Part print with two shaded views. Sizes in mm from the minimum x, y, z corner. A direction names the side the tool comes from. Give positions to 0.01 mm unless a question says otherwise; leave off trailing zeros. Write each loop counter-clockwise with the first axis right and the second up, starting at its lowest first coordinate (ties: lowest second). Pieces come first, ordered by that corner, then holes. Notation, with made-up numbers: (73.5, 71) -> (94.5, 71) arc R20 cw to (94.5, 104) -> close; hole circle Ø6 at (74, -37). An arc over 180 degrees is marked (long way). Write item = value, one per line. Start each with the question number.
Q1. Wall check: line 1 (Y direction, x = 4, z = 24.5); line 2 (Z direction, x = 14.25, y = 8); line 3 (Z direction, x = 22.25, y = 31). Give the ranges that are in metal, low to high.
Q2. Saw through at A-A, the plane x = 4. List the corners of the cut face in (y, z).
Q3. Saw through at C-C, the plane z = 4.25. List the corners of the cut face in (x, y), then the cut area to 3 significant figures.
Q4. Mould opens along Y. For the marked faces 4, 5, 6 and 7 say: pulls with the +Y half, pulls with the -Y half, needs draft (parallel to the pull), parting line crosses it, or undercut.
Q5. Tool access for the marked faces 1, 2 and 3: list every direction of +Z, -Z, +X, -X, +Y, -Y with a clear straight run to the whole face (end or side of a thin tool).
Q6. Drop flat-ended pins along their axis: P1, Ø10, axis at x = 11.5, z = 19, coming from the +Y side; P2, Ø6.5, axis at x = 8, z = 24.5, coming from the -Y side; P3, Ø8, axis at y = 14, z = 9.5, coming from the -X side; P4, Ø2, axis at x = 24.5, y = 18, coming from the -Z side. Give the stop position or say it passes through.
Q7. Saw through at B-B, the plane y = 20.5. List the corners of the cut face in (x, z).
Q8. Saw through at D-D, the plane z = 21.5. List the corners of the cut face in (x, y), then the cut area to 3 significant figures.
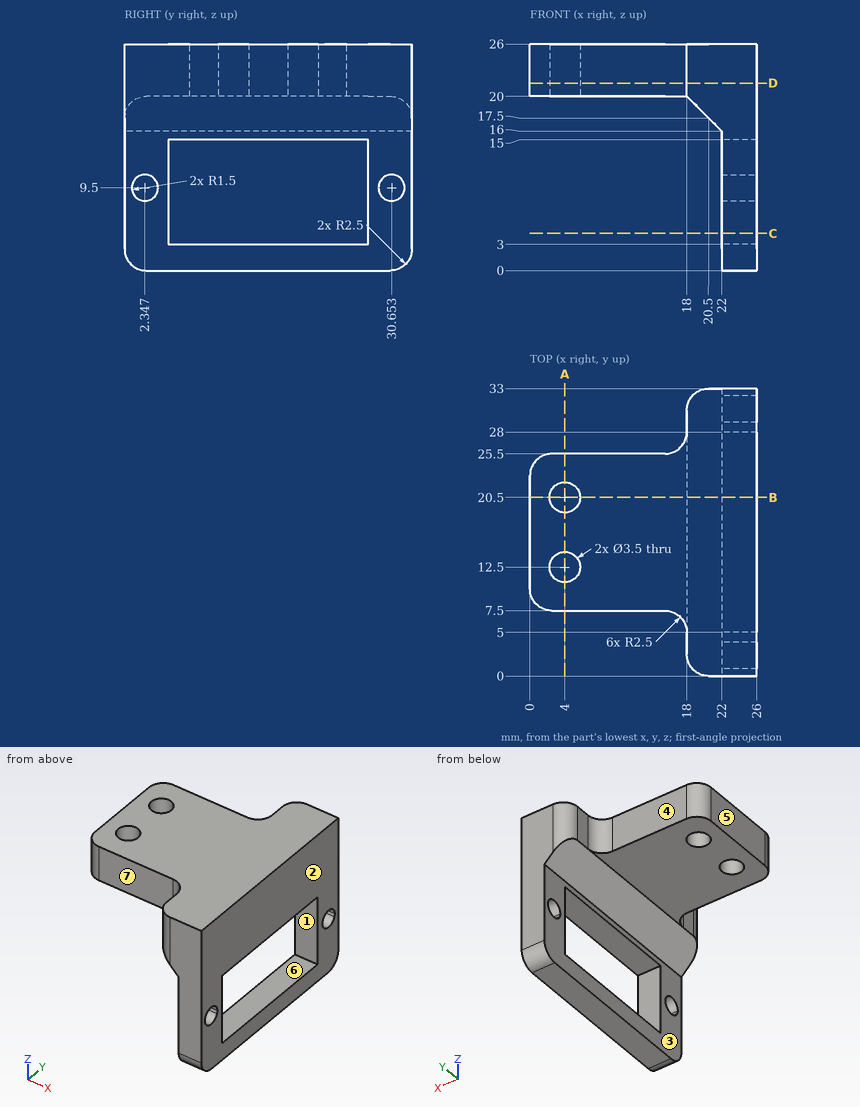
Report:
q1.line_1 = 7.5 to 10.75, 14.25 to 18.75, 22.25 to 25.5
q1.line_2 = 20 to 26
q1.line_3 = 0.05 to 8.04, 10.96 to 26
q2.outline = (7.5, 20) -> (10.75, 20) -> (10.75, 26) -> (7.5, 26) -> close; (14.25, 20) -> (18.75, 20) -> (18.75, 26) -> (14.25, 26) -> close; (22.25, 20) -> (25.5, 20) -> (25.5, 26) -> (22.25, 26) -> close
q3.outline = (22, 0) -> (26, 0) -> (26, 5) -> (22, 5) -> close; (22, 28) -> (26, 28) -> (26, 33) -> (22, 33) -> close
q3.area = 40.0 mm2
q4.face_4 = pulls with the +Y half
q4.face_5 = needs draft
q4.face_6 = undercut
q4.face_7 = pulls with the -Y half
q5.face_1 = +X, -X
q5.face_2 = +Z, -Z, +X, +Y, -Y
q5.face_3 = -Z, -X, +Y, -Y
q6.P1 = 25.67
q6.P2 = 7.5
q6.P3 = through
q6.P4 = 0
q7.outline = (0, 20) -> (2.25, 20) -> (2.25, 26) -> (0, 26) -> close; (5.75, 20) -> (18, 20) -> (22, 16) -> (22, 15) -> (26, 15) -> (26, 26) -> (5.75, 26) -> close; (22, 0) -> (26, 0) -> (26, 3) -> (22, 3) -> close
q8.outline = (0, 10) arc R2.5 ccw to (2.5, 7.5) -> (15.5, 7.5) arc R2.5 cw to (18, 5) -> (18, 2.5) arc R2.5 ccw to (20.5, 0) -> (26, 0) -> (26, 33) -> (20.5, 33) arc R2.5 ccw to (18, 30.5) -> (18, 28) arc R2.5 cw to (15.5, 25.5) -> (2.5, 25.5) arc R2.5 ccw to (0, 23) -> close; hole circle Ø3.5 at (4, 12.5); hole circle Ø3.5 at (4, 20.5)
q8.area = 566 mm2
